Check sheet for the modelled part. Datum: model origin and axes. Units: mm. Coordinates: 2 decimals unless noted, no trailing zeros. Loops run counter-clockwise (first coordinate to the right, second up) from the corner with the lowest first, then second, coordinate; pieces in that order, holes last.
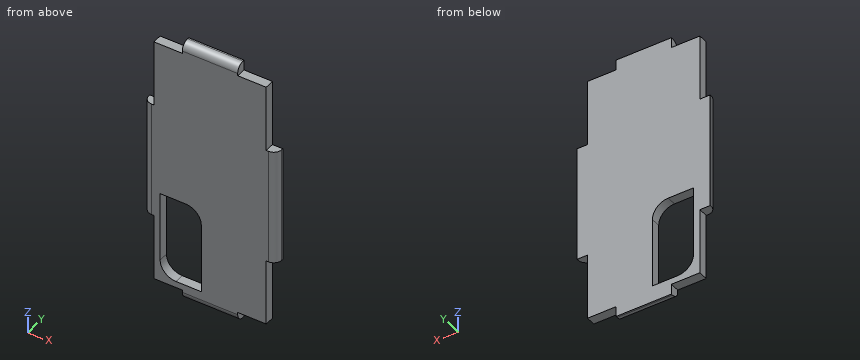
```python
from build123d import *

# Parameters (mm, degrees)
F0_W     = 42
F0_H     = 85
F1_DEPTH = 3
F2_R     = 3
F4_DEPTH = 3
F5_W     = 13
F5_H     = 27
F6_DEPTH = 3
F7_R     = 5
F8_R     = 2.5


with BuildPart() as f1:
    # F0 (on Front) → F1 (new body)
    with BuildSketch(Plane.XZ):
        with Locations((-12.290565, -9.565399)):
            Rectangle(F0_W, F0_H)
    extrude(amount=F1_DEPTH)

    # F2
    f2_edges = [f1.edges().sort_by_distance(p)[0] for p in [
        (-33.290565, -1.5, 32.934601),
        (8.709435, -1.5, 32.934601),
        (8.709435, -1.5, -52.065399),
        (-33.290565, -1.5, -52.065399),
    ]]
    fillet(f2_edges, radius=F2_R)

    # F3 (on face) → F4 (cut, through all)
    with BuildSketch(Plane(origin=(0, 0, 0), x_dir=(-1, 0, 0), z_dir=(0, 1, 0))):
        with BuildLine():
            Line((-5.459435, 8.759601), (-5.459435, 29.684601))
            Line((-5.459435, 29.684601), (3.540565, 29.684601))
            Line((3.540565, 29.684601), (3.540565, 32.934601))
            Line((3.540565, 32.934601), (-5.709435, 32.934601))
            ThreePointArc((-5.709435, 32.934601), (-7.830755, 32.055922), (-8.709435, 29.934601))
            Line((-8.709435, 29.934601), (-8.709435, 8.759601))
            Line((-8.709435, 8.759601), (-5.459435, 8.759601))
        make_face()
        with BuildLine():
            Line((21.040565, 32.934601), (21.040565, 29.684601))
            Line((21.040565, 29.684601), (30.040565, 29.684601))
            Line((30.040565, 29.684601), (30.040565, 8.759601))
            Line((30.040565, 8.759601), (33.290565, 8.759601))
            Line((33.290565, 8.759601), (33.290565, 29.934601))
            ThreePointArc((33.290565, 29.934601), (32.411885, 32.055922), (30.290565, 32.934601))
            Line((30.290565, 32.934601), (21.040565, 32.934601))
        make_face()
        with BuildLine():
            Line((33.290565, -27.890399), (30.040565, -27.890399))
            Line((30.040565, -27.890399), (30.040565, -48.815399))
            Line((30.040565, -48.815399), (21.040565, -48.815399))
            Line((21.040565, -48.815399), (21.040565, -52.065399))
            Line((21.040565, -52.065399), (30.290565, -52.065399))
            ThreePointArc((30.290565, -52.065399), (32.411885, -51.186719), (33.290565, -49.065399))
            Line((33.290565, -49.065399), (33.290565, -27.890399))
        make_face()
        with BuildLine():
            Line((-5.459435, -48.815399), (-5.459435, -27.890399))
            Line((-5.459435, -27.890399), (-8.709435, -27.890399))
            Line((-8.709435, -27.890399), (-8.709435, -49.065399))
            ThreePointArc((-8.709435, -49.065399), (-7.830755, -51.186719), (-5.709435, -52.065399))
            Line((-5.709435, -52.065399), (3.540565, -52.065399))
            Line((3.540565, -52.065399), (3.540565, -48.815399))
            Line((3.540565, -48.815399), (-5.459435, -48.815399))
        make_face()
    extrude(amount=-F4_DEPTH, mode=Mode.SUBTRACT)

    # F5 (on face) → F6 (cut, through all)
    with BuildSketch(Plane.XZ.offset(3)):
        with Locations((-21.540565, -33.315399)):
            Rectangle(F5_W, F5_H)
    extrude(amount=-F6_DEPTH, mode=Mode.SUBTRACT)

    # F7
    f7_edges = [f1.edges().sort_by_distance(p)[0] for p in [
        (-15.040565, -1.5, -19.815399),
        (-28.040565, -1.5, -46.815399),
    ]]
    fillet(f7_edges, radius=F7_R)

    # F8
    f8_edges = [f1.edges().sort_by_distance(p)[0] for p in [
        (-12.290565, -3, 32.934601),
        (8.709435, -3, -9.565399),
        (-12.290565, -3, -52.065399),
        (-33.290565, -3, -9.565399),
    ]]
    fillet(f8_edges, radius=F8_R)


solid = f1.part
```
1) Depth check by flat-ended pin: pin 1 (1.5 mm diameter, centred on x = -19.5, y = -1.5, fed in from +Z); pin 2 (0.9 mm diameter, centred on x = 1.5, y = -1, fed in from +Z); pin 3 (0.9 mm diameter, centred on x = 6.5, y = -1, fed in from -Z). Enter the tip coordinate at first touch or a pass-through.
Answer sheet:
pin 1: stops at z = 32.92
pin 2: stops at z = 29.68
pin 3: stops at z = -27.89
2) Section check B-B on y = -2.45. Enter the section's corners in (x, z).
Answer sheet:
outline: (-32.36, -27.89) - (-30.04, -27.89) - (-30.04, -48.82) - (-21.04, -48.82) - (-21.04, -51.13) - (-3.54, -51.13) - (-3.54, -48.82) - (5.46, -48.82) - (5.46, -27.89) - (7.77, -27.89) - (7.77, 8.76) - (5.46, 8.76) - (5.46, 29.68) - (-3.54, 29.68) - (-3.54, 32) - (-21.04, 32) - (-21.04, 29.68) - (-30.04, 29.68) - (-30.04, 8.76) - (-32.36, 8.76) - close; hole (-28.04, -41.82) arc R5 ccw to (-23.04, -46.82) - (-15.04, -46.82) - (-15.04, -24.82) arc R5 ccw to (-20.04, -19.82) - (-28.04, -19.82) - close
3) Section check A-A on z = -26. Enter the section's corners in (x, y).
Answer sheet:
outline: (-33.29, -0.5) arc R2.5 ccw to (-30.79, -3) - (-28.04, -3) - (-28.04, 0) - (-33.29, 0) - close; (-15.04, -3) - (6.21, -3) arc R2.5 ccw to (8.71, -0.5) - (8.71, 0) - (-15.04, 0) - close
4) Section check C-C on x = -16. Enter the section's corners in (y, z), plus the area to 3 significant figures.
Answer sheet:
outline: (-3, -49.57) arc R2.5 ccw to (-0.5, -52.07) - (0, -52.07) - (0, -46.82) - (-3, -46.82) - close; (-3, -21.87) - (0, -21.87) - (0, 32.93) - (-0.5, 32.93) arc R2.5 ccw to (-3, 30.43) - close
area: 177 mm2
5) Scan lines: line 1 (X direction, y = -0.35, z = -40.5); line 2 (Z direction, x = -23, y = -1.2); line 3 (Z direction, x = -21, y = -0.1). Record each from-to range of solid material in increasing order.
Answer sheet:
line 1: x = -30.04 to -28.04, -15.04 to 5.46
line 2: z = -48.82 to -46.82, -19.82 to 29.68
line 3: z = -52.07 to -46.82, -19.82 to 32.93
6) Section check D-D on z = -5. Enter the section's corners in (x, y), plus the area to 3 significant figures.
Answer sheet:
outline: (-33.29, -0.5) arc R2.5 ccw to (-30.79, -3) - (6.21, -3) arc R2.5 ccw to (8.71, -0.5) - (8.71, 0) - (-33.29, 0) - close
area: 123 mm2
